Here's how the part is built. I have some questions about the finished solid (model axes, mm). Coordinates: 2 decimals unless noted, no trailing zeros. Write each loop counter-clockwise with the first axis right and the second up, starting at its lowest first coordinate (ties: lowest second). Pieces come first, ordered by that corner, then holes. Notation, with made-up numbers: (31.25, 4.25) - (82.25, 4.25) arc R17 cw to (82.25, 18.25) - close; hole circle Ø6 at (53, 53). An arc over 180 degrees is marked (long way). Answer in a Markdown table with one row per item. Add a question column.
Item 1: Imagine slicing it at A-A (x = 14). Please give me the cut outline in (y, z) (3 decimals).
Item 2: Imagine slicing it at C-C (y = -0.75). Please give me the cut outline in (x, z) (3 decimals), plus the area to 3 significant figures.
Item 3: We'd pull the mould along Z, two halves only. Please class faces 1 (the face through (-13.343, 1.041, -28.658)), 2 (the face through (-25.4, 3, -28)), 3 (the face through (0, 2, -34.925)): +Z half, -Z half, draft (parallel to the pull), parting line (faces both ways), or undercut.
Item 4: Imagine slicing it at D-D (x = -15.24). Please give me the cut outline in (y, z) (3 decimals), plus the area to 3 significant figures.
Item 5: If I drill on probe 1 along Z at (x, y) = (15.24, -0.5) (3 decimals); probe 2 along X at (y, z) = (1, -29.5); probe 3 along X at (y, z) = (2, -27.25), over which ranges is the centre line in solid material (lowest first)? Write a range as from..to.
Item 6: Imagine slicing it at B-B (z = -24.75). Please give me the cut outline in (x, y) (3 decimals).
Item 7: I'm going to push a flat-ended pin straight in: pin 1 (4 mm diameter, centred on x = -2, z = -32, fed in from -Y). Where does the tip first touch, or does it pass through?
from build123d import *
from build123d.topology import SkipClean

# Parameters (mm, degrees)
SKETCH1_W              = 50.8
SKETCH1_H              = 44.45
BOSS_EXTRUDE1_DEPTH    = 6.35
BOSS_EXTRUDE2_DEPTH    = 44.45
M4X0_7_TAPPED_HOLE1_D  = 3.3
BOSS_EXTRUDE3_DEPTH    = 12.7
F_10_24_TAPPED_HOLE1_D = 3.7973
SKETCH10_W             = 50.8
SKETCH10_H             = 44.45
CUT_EXTRUDE1_DEPTH     = 25.4


with BuildPart() as part:
    # Sketch1 → Boss-Extrude1 (new body)
    with BuildSketch(Plane(origin=(0, 0, 0), x_dir=(1, 0, 0), z_dir=(0, 1, 0))):
        Rectangle(SKETCH1_W, SKETCH1_H)
    extrude(amount=BOSS_EXTRUDE1_DEPTH)

    # Sketch2 → Boss-Extrude2 (add)
    with BuildSketch(Plane.XY.offset(22.225)):
        with BuildLine():
            Line((-25.4, 0), (25.4, 0))
            ThreePointArc((25.4, 0), (0, -5.608040792), (-25.4, 0))
        make_face()
    extrude(amount=-BOSS_EXTRUDE2_DEPTH)

    # M4x0.7 Tapped Hole1 (through all)
    with Locations(Plane(origin=(0, 6.35, 0), x_dir=(1, 0, 0), z_dir=(0, 1, 0))):
        with Locations((0, 14.6499912), (-17.9500022, -14.6500088), (17.9499978, -14.6500088)):
            Hole(M4X0_7_TAPPED_HOLE1_D / 2)

    # Sketch6 → Boss-Extrude3 (add)
    with SkipClean():  # the faces are left unmerged after this step: merging them gives an invalid solid
        with BuildSketch(Plane(origin=(0, 0, -22.225), x_dir=(-1, 0, 0), z_dir=(0, 0, -1))):
            with BuildLine():
                Line((-25.4, 6.35), (25.4, 6.35))
                Line((25.4, 6.35), (25.4, 0))
                ThreePointArc((25.4, 0), (0, -5.608040792), (-25.4, 0))
                Line((-25.4, 0), (-25.4, 6.35))
            make_face()
        extrude(amount=BOSS_EXTRUDE3_DEPTH)

    # #10-24 Tapped Hole1 (through all)
    with Locations(Plane(origin=(0, 6.35, 0), x_dir=(1, 0, 0), z_dir=(0, 1, 0))):
        with Locations((-15.24, 28.575), (15.24, 28.575)):
            Hole(F_10_24_TAPPED_HOLE1_D / 2)

    # Sketch10 → Cut-Extrude1 (cut)
    with BuildSketch(Plane(origin=(0, 6.35, 0), x_dir=(1, 0, 0), z_dir=(0, 1, 0))):
        Rectangle(SKETCH10_W, SKETCH10_H)
    extrude(amount=-CUT_EXTRUDE1_DEPTH, mode=Mode.SUBTRACT)


solid = part.part
Here are the results:
| question | item | result |
|---|---|---|
| 1 | outline | (-3.961, -34.925) - (6.35, -34.925) - (6.35, -30.013) - (-3.961, -30.013) - close; (-3.961, -27.137) - (6.35, -27.137) - (6.35, -22.225) - (-3.961, -22.225) - close |
| 2 | outline | (-23.718, -34.925) - (23.718, -34.925) - (23.718, -22.225) - (-23.718, -22.225) - close; hole circle Ø3.797 at (-15.24, -28.575); hole circle Ø3.797 at (15.24, -28.575) |
| 2 | area | 580 mm2 |
| 3 | face 1 | undercut |
| 3 | face 2 | draft |
| 3 | face 3 | -Z half |
| 4 | outline | (-3.651, -34.925) - (6.35, -34.925) - (6.35, -30.474) - (-3.651, -30.474) - close; (-3.651, -26.676) - (6.35, -26.676) - (6.35, -22.225) - (-3.651, -22.225) - close |
| 4 | area | 89.0 mm2 |
| 5 | probe 1 | z = -34.925..-30.474, -26.676..-22.225 |
| 5 | probe 2 | x = -25.4..-16.9, -13.58..13.58, 16.9..25.4 |
| 5 | probe 3 | x = -25.4..-16.6, -13.88..13.88, 16.6..25.4 |
| 6 | outline | (-25.4, 0) arc R60.325 ccw to (25.4, 0) - (25.4, 6.35) - (-25.4, 6.35) - close |
| 7 | pin 1 | stops at y = -5.61 |
